Design review of the part built by this model. Coordinates are the model's own, in mm. A direction names the side the tool comes from. Give positions to 0.01 mm unless a question says otherwise; leave off trailing zeros. Loops run counter-clockwise (first coordinate to the right, second up) from the corner with the lowest first, then second, coordinate; pieces in that order, holes last. Notation, with made-up numbers: (4, 48) - (28, 48) arc R6 cw to (28, 55) - close; hole circle Ø8 at (52.5, 27.25). An arc over 180 degrees is marked (long way). Put each result on its own line as item: value. Start each with the question number.
```python
from build123d import *

# Parameters (mm, degrees)
BASEFLANGE_W                   = 715
BASEFLANGE_H                   = 50
BASE_FLANGE1_DEPTH             = 2
EDGE_FLANGE1_STRIP_W           = 10
EDGE_FLANGE1_STRIP_H           = 2
EDGE_FLANGE1_STRIP_CUT_DEPTH   = 715
EDGE_FLANGE1_STRIP_2_W         = 10
EDGE_FLANGE1_STRIP_2_H         = 2
EDGE_FLANGE1_STRIP_CUT_2_DEPTH = 715
EDGE_FLANGE1_DEPTH             = 715
EDGE_FLANGE1_BEND_DEPTH        = 715
EDGE_FLANGE2_STRIP_W           = 10
EDGE_FLANGE2_STRIP_H           = 2
EDGE_FLANGE2_STRIP_CUT_DEPTH   = 715
EDGE_FLANGE2_STRIP_2_W         = 10
EDGE_FLANGE2_STRIP_2_H         = 2
EDGE_FLANGE2_STRIP_CUT_2_DEPTH = 715
EDGE_FLANGE2_DEPTH             = 715
EDGE_FLANGE2_BEND_DEPTH        = 715


# Sheet-metal steps are written as plain solids
with BuildPart() as part:
    # BaseFlange → Base-Flange1 (new body)
    with BuildSketch(Plane.XY):
        Rectangle(BASEFLANGE_W, BASEFLANGE_H)
    extrude(amount=BASE_FLANGE1_DEPTH)

    # Edge-Flange1 strip (across the edge) → Edge-Flange1 strip cut (cut)
    with BuildSketch(Plane(origin=(357.5, 25, 2), x_dir=(0, -1, 0), z_dir=(-1, 0, 0))):
        with Locations((-2, -1)):
            Rectangle(EDGE_FLANGE1_STRIP_W, EDGE_FLANGE1_STRIP_H)
    extrude(amount=EDGE_FLANGE1_STRIP_CUT_DEPTH, mode=Mode.SUBTRACT)

    # Edge-Flange1 strip 2 (across the edge) → Edge-Flange1 strip cut 2 (cut)
    with BuildSketch(Plane(origin=(-357.5, -25, 2), x_dir=(0, 1, 0), z_dir=(1, 0, 0))):
        with Locations((-2, -1)):
            Rectangle(EDGE_FLANGE1_STRIP_2_W, EDGE_FLANGE1_STRIP_2_H)
    extrude(amount=EDGE_FLANGE1_STRIP_CUT_2_DEPTH, mode=Mode.SUBTRACT)

    # Edge-Flange1 section (across the edge) → Edge-Flange1 (add)
    with BuildSketch(Plane(origin=(357.5, 25, 2), x_dir=(0, -1, 0), z_dir=(-1, 0, 0))):
        with BuildLine():
            Line((0, 1), (0, 20))
            Line((0, 20), (2, 20))
            Line((2, 20), (2, 1))
            ThreePointArc((2, 1), (2.292893219, 0.292893219), (3, 0))
            Line((3, 0), (3, -2))
            ThreePointArc((3, -2), (0.878679656, -1.121320344), (0, 1))
        make_face()
    extrude(amount=EDGE_FLANGE1_DEPTH)

    # Edge-Flange1 section 2 (across the edge) → Edge-Flange1 bend (add)
    with BuildSketch(Plane(origin=(-357.5, -25, 2), x_dir=(0, 1, 0), z_dir=(1, 0, 0))):
        with BuildLine():
            Line((0, 1), (0, 20))
            Line((0, 20), (2, 20))
            Line((2, 20), (2, 1))
            ThreePointArc((2, 1), (2.292893219, 0.292893219), (3, 0))
            Line((3, 0), (3, -2))
            ThreePointArc((3, -2), (0.878679656, -1.121320344), (0, 1))
        make_face()
    extrude(amount=EDGE_FLANGE1_BEND_DEPTH)

    # Edge-Flange2 strip (across the edge) → Edge-Flange2 strip cut (cut)
    with BuildSketch(Plane(origin=(357.5, 23, 22), x_dir=(0, 0, -1), z_dir=(-1, 0, 0))):
        with Locations((-2, -1)):
            Rectangle(EDGE_FLANGE2_STRIP_W, EDGE_FLANGE2_STRIP_H)
    extrude(amount=EDGE_FLANGE2_STRIP_CUT_DEPTH, mode=Mode.SUBTRACT)

    # Edge-Flange2 strip 2 (across the edge) → Edge-Flange2 strip cut 2 (cut)
    with BuildSketch(Plane(origin=(-357.5, -23, 22), x_dir=(0, 0, -1), z_dir=(1, 0, 0))):
        with Locations((-2, -1)):
            Rectangle(EDGE_FLANGE2_STRIP_2_W, EDGE_FLANGE2_STRIP_2_H)
    extrude(amount=EDGE_FLANGE2_STRIP_CUT_2_DEPTH, mode=Mode.SUBTRACT)

    # Edge-Flange2 section (across the edge) → Edge-Flange2 (add)
    with BuildSketch(Plane(origin=(357.5, 23, 22), x_dir=(0, 0, -1), z_dir=(-1, 0, 0))):
        with BuildLine():
            Line((0, 1), (0, 8))
            Line((0, 8), (2, 8))
            Line((2, 8), (2, 1))
            ThreePointArc((2, 1), (2.292893219, 0.292893219), (3, 0))
            Line((3, 0), (3, -2))
            ThreePointArc((3, -2), (0.878679656, -1.121320344), (0, 1))
        make_face()
    extrude(amount=EDGE_FLANGE2_DEPTH)

    # Edge-Flange2 section 2 (across the edge) → Edge-Flange2 bend (add)
    with BuildSketch(Plane(origin=(-357.5, -23, 22), x_dir=(0, 0, -1), z_dir=(1, 0, 0))):
        with BuildLine():
            Line((0, 1), (0, 8))
            Line((0, 8), (2, 8))
            Line((2, 8), (2, 1))
            ThreePointArc((2, 1), (2.292893219, 0.292893219), (3, 0))
            Line((3, 0), (3, -2))
            ThreePointArc((3, -2), (0.878679656, -1.121320344), (0, 1))
        make_face()
    extrude(amount=EDGE_FLANGE2_BEND_DEPTH)


solid = part.part
```
Item 1: Machinability: for faces 5 (the flat face through (5, 23, 11)), 6 (the flat face through (-5, 0, 0)), which of the approach directions +Z, -Z, +X, -X, +Y, -Y give a long, thin tool a straight path to every point of the face, cutting with its end or side? Answer none if there is none.
Item 2: Mouldability with a two-part tool opening along Y and no side actions: class faces 1 (the flat face through (357.5, -2, 1)), 2 (the flat face through (-5, -25, 11)), 3 (the flat face through (-5, -23, 11)), 4 (the flat face through (-5, 0, 2)) as pulls with the +Y half, pulls with the -Y half, needs draft (parallel to the pull), parting line crosses it, or undercut.
Item 3: For P1, Ø2, axis at x = -135, z = 21, coming from the +Y side; P2, Ø1.5, axis at x = 82, y = 4.5, coming from the +Z side; P3, Ø0.6, axis at x = -5.5, z = 20.5, coming from the -Y side, all flat-tipped, find the tip position at first contact; note any pin that passes through.
Item 4: Consider section B-B (x = 191.5). State the section outline as (y, z) points.
Item 5: For L1, parallel to Y at x = -134, z = 11.75; L2, parallel to Z at x = -162, y = -18.5; L3, parallel to Z at x = -255, y = 14.5, list the stretches that pass through material, from the lowest coordinate up. Write a range as from..to.
Item 6: Consider section A-A (z = 10.75). State the section outline as (x, y) points, plus the area to 3 significant figures.
Item 7: Consider section C-C (y = 5). State the section outline as (x, z) points, plus the area to 3 significant figures.
Geometry says:
1. face 5: +X, -X
1. face 6: -Z, +X, -X, +Y, -Y
2. face 1: needs draft
2. face 2: pulls with the -Y half
2. face 3: undercut
2. face 4: undercut
3. P1: stops at y = 24.83
3. P2: stops at z = 2
3. P3: stops at y = -24.75
4. outline: (-25, 3) arc R3 ccw to (-22, 0) - (22, 0) arc R3 ccw to (25, 3) - (25, 19) arc R3 ccw to (22, 22) - (15, 22) - (15, 20) - (22, 20) arc R1 cw to (23, 19) - (23, 3) arc R1 cw to (22, 2) - (-22, 2) arc R1 cw to (-23, 3) - (-23, 19) arc R1 cw to (-22, 20) - (-15, 20) - (-15, 22) - (-22, 22) arc R3 ccw to (-25, 19) - close
5. L1: y = -25..-23, 23..25
5. L2: z = 0..2, 20..22
5. L3: z = 0..2
6. outline: (-357.5, -25) - (357.5, -25) - (357.5, -23) - (-357.5, -23) - close; (-357.5, 23) - (357.5, 23) - (357.5, 25) - (-357.5, 25) - close
6. area: 2,860 mm2
7. outline: (-357.5, 0) - (357.5, 0) - (357.5, 2) - (-357.5, 2) - close
7. area: 1,430 mm2
